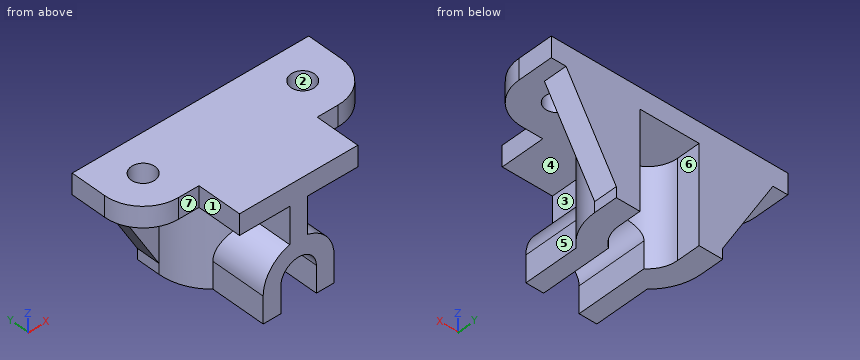
from build123d import *

# Parameters (mm, degrees)
SKETCH_1_R           = 4
EXTRUDE_1_DEPTH      = 7
EXTRUDE_2_DEPTH      = 33
EXTRUDE_3_DEPTH      = 8
EXTRUDE_4_REACH      = 71.282
EXTRUDE_4_END_RADIUS = 18
CUT_EXTRUDE_1_DEPTH  = 70.28203236


with BuildPart() as part:
    # 草图1 → 凸台-拉伸1 (new body)
    with BuildSketch(Plane.XY):
        with BuildLine():
            Line((-40, 0), (40, 0))
            Line((40, 0), (40, -12))
            ThreePointArc((40, -12), (36.192388155, -21.192388155), (27, -25))
            Line((27, -25), (20, -25))
            Line((20, -25), (20, -40))
            Line((20, -40), (-20, -40))
            Line((-20, -40), (-20, -25))
            Line((-20, -25), (-27, -25))
            ThreePointArc((-27, -25), (-36.192388155, -21.192388155), (-40, -12))
            Line((-40, -12), (-40, 0))
        make_face()
        with Locations((-27, -12)):
            Circle(SKETCH_1_R, mode=Mode.SUBTRACT)
        with Locations(Location((27, -12, 0), (0, 0, 180))):
            Circle(SKETCH_1_R, mode=Mode.SUBTRACT)
    extrude(amount=-EXTRUDE_1_DEPTH)

    # 草图2 → 凸台-拉伸2 (add)
    with BuildSketch(Plane(origin=(0, 0, -7), x_dir=(-1, 0, 0), z_dir=(0, 0, -1))):
        with BuildLine():
            Line((-10, 0), (-10, -8))
            ThreePointArc((-10, -8), (0, -18), (10, -8))
            Line((10, -8), (10, 0))
            Line((10, 0), (18, 0))
            Line((18, 0), (18, -8))
            ThreePointArc((18, -8), (0, -26), (-18, -8))
            Line((-18, -8), (-18, 0))
            Line((-18, 0), (-10, 0))
        make_face()
    extrude(amount=EXTRUDE_2_DEPTH)

    # 草图3 → 凸台-拉伸3 (add)
    with BuildSketch(Plane(origin=(0, 0, 0), x_dir=(1, 0, 0), z_dir=(0, 1, 0))):
        Polygon((18, 36.444863729), (35, 7), (18, 7), align=None)
        Polygon((-18, 36.444863729), (-35, 7), (-18, 7), align=None)
    extrude(amount=-EXTRUDE_3_DEPTH)

    # 凸台-拉伸4: up to this cylinder (the profile starts outside it)
    extrude_4_end = Plane(origin=(0, -8, -28.116235), z_dir=(0, 0, 1)) * Cylinder(EXTRUDE_4_END_RADIUS, 179.564, mode=Mode.PRIVATE)
    # 草图4 → 凸台-拉伸4 (add, up to the surface)
    with BuildSketch(Plane.XZ.offset(40), mode=Mode.PRIVATE) as extrude_4_sk1:
        with BuildLine():
            Line((12, -40), (12, -31))
            ThreePointArc((12, -31), (9.486832981, -23.651530772), (3, -19.381049961))
            Line((3, -19.381049961), (3, -7))
            Line((3, -7), (-3, -7))
            Line((-3, -7), (-3, -19.381049961))
            ThreePointArc((-3, -19.381049961), (-9.486832981, -23.651530772), (-12, -31))
            Line((-12, -31), (-12, -40))
            Line((-12, -40), (12, -40))
        make_face()
    extrude_4_tool1 = extrude(extrude_4_sk1.sketch, amount=-EXTRUDE_4_REACH, mode=Mode.PRIVATE) - extrude_4_end
    add(extrude_4_tool1.solids().sort_by_distance((0, -40, -28.116235))[0])

    # 草图5 → 切除-拉伸1 (cut, through all)
    with BuildSketch(Plane.XZ.offset(40)):
        with BuildLine():
            Line((6, -40), (6, -31))
            ThreePointArc((6, -31), (0, -25), (-6, -31))
            Line((-6, -31), (-6, -40))
            Line((-6, -40), (6, -40))
        make_face()
    extrude(amount=-CUT_EXTRUDE_1_DEPTH, mode=Mode.SUBTRACT)


solid = part.part
Read the model definition and answer for the solid it produces. Units are mm, in the model's axes. Face numbers are marked on the shaded views. A direction names the side the tool comes from. Give positions to 0.01 mm unless a question says otherwise; leave off trailing zeros. Write each loop counter-clockwise with the first axis right and the second up, starting at its lowest first coordinate (ties: lowest second). Pieces come first, ordered by that corner, then holes. Notation, with made-up numbers: (59, -2) - (96, -2) arc R33 ccw to (96, 26) - close; hole circle Ø4 at (9, 10). An arc over 180 degrees is marked (long way). Answer in a Markdown table with one row per item. Add a question column.
Item 1: Section B-B, the plane y = -31.5 is taken. Write down the section's boundary in (x, z).
Item 2: Determine the mould class of the marked faces 1, 2 and 3 for opening direction X: pulls with the +X half, pulls with the -X half, needs draft (parallel to the pull), parting line crosses it, or undercut.
Item 3: Section A-A, the plane z = -3 is taken. Write down the section's boundary in (x, y), and give its area (3 significant figures).
Item 4: Section C-C, the plane z = -32 is taken. Write down the section's boundary in (x, y), and give its area (3 significant figures).
Item 5: Flat-ended cylindrical pins translate along their axes: P1, Ø4.5, axis at y = -30, z = -37, coming from the -X side; P2, Ø13.5, axis at y = -29.5, z = -14.5, coming from the -X side; P3, Ø3, axis at y = -6, z = -39, coming from the -X side. Find the tip coordinate at first contact, or state that the pin passes through.
Item 6: Section D-D, the plane x = 0 is taken. Write down the section's boundary in (y, z).
Item 7: A tool of negligible diameter and unlimited length cuts with its end or side. For the marked faces 4, 5, 6 and 7, from which of +Z, -Z, +X, -X, +Y, -Y can it reach the whole face along a straight path? Write none if from no direction.
Item 8: Find the intervals of material crossed by L1, parallel to X at y = -12, z = -2.5; L2, parallel to Y at x = 27, z = -1; L3, parallel to X at y = -11, z = -4.5, in increasing order.
Recorded:
| question | item | result |
|---|---|---|
| 1 | outline | (-20, -7) - (-3, -7) - (-3, -19.38) arc R12 ccw to (-12, -31) - (-12, -40) - (-6, -40) - (-6, -31) arc R6 cw to (6, -31) - (6, -40) - (12, -40) - (12, -31) arc R12 ccw to (3, -19.38) - (3, -7) - (20, -7) - (20, 0) - (-20, 0) - close |
| 2 | face 1 | pulls with the -X half |
| 2 | face 2 | undercut |
| 2 | face 3 | pulls with the +X half |
| 3 | outline | (-40, -12) arc R13 ccw to (-27, -25) - (-20, -25) - (-20, -40) - (20, -40) - (20, -25) - (27, -25) arc R13 ccw to (40, -12) - (40, 0) - (-40, 0) - close; hole circle Ø8 at (-27, -12); hole circle Ø8 at (27, -12) |
| 3 | area | 2,430 mm2 |
| 4 | outline | (-20.57, -8) - (-18, -8) arc R18 ccw to (-12, -21.42) - (-12, -40) - (-6, -40) - (-6, -16) arc R10 cw to (-10, -8) - (-10, 0) - (-20.57, 0) - close; (6, -40) - (12, -40) - (12, -21.42) arc R18 ccw to (18, -8) - (20.57, -8) - (20.57, 0) - (10, 0) - (10, -8) arc R10 cw to (6, -16) - close |
| 4 | area | 620 mm2 |
| 5 | P1 | stops at x = -12 |
| 5 | P2 | stops at x = -10.32 |
| 5 | P3 | stops at x = -18 |
| 6 | outline | (-40, -25) - (-18, -25) - (-18, -7) - (0, -7) - (0, 0) - (-40, 0) - close |
| 7 | face 4 | +X, -Y |
| 7 | face 5 | -Z, +X, -Y |
| 7 | face 6 | -Z, +Y |
| 7 | face 7 | +Z, -Z, -X, -Y |
| 8 | L1 | x = -40 to -31, -23 to 23, 31 to 40 |
| 8 | L2 | y = -25 to -16, -8 to 0 |
| 8 | L3 | x = -40 to -30.87, -23.13 to 23.13, 30.87 to 40 |
